Part model, mm, in its own coordinate system. A direction names the side the tool comes from. Give positions to 0.01 mm unless a question says otherwise; leave off trailing zeros. Write each loop counter-clockwise with the first axis right and the second up, starting at its lowest first coordinate (ties: lowest second). Pieces come first, ordered by that corner, then holes. Notation, with made-up numbers: M 48.25,-16 L 80.25,-16 A12 ccw 80.25,0 Z; hole C 36.5,5 d8. An arc over 180 degrees is marked long. Use CSV: the item, a comma, the result in double quotes. Start each with the question number.
1. Mould opens along Y. For faces 4 (the face through (28.71, -7.103, 0.035)), 5 (the face through (-57.15, -76.99, 0.04)), 6 (the face through (-36, -21, 27.5)) say: pulls with the +Y half, pulls with the -Y half, needs draft (parallel to the pull), parting line crosses it, or undercut.
2. Band-saw the part on C-C, the plane y = -9. List the corners of the cut face in (x, z), then the cut area to 3 significant figures.
3. Drop flat-ended pins along their axis: pin 1 Ø2 at (x, z) = (-40.5, -5) entering from -Y; pin 2 Ø5.5 at (x, z) = (-45.5, -13) entering from +Y; pin 3 Ø9 at (x, z) = (43, -10.5) entering from -Y; pin 4 Ø3.5 at (y, z) = (-59.32, -14.5) entering from -X. Give the stop position or say it passes through.
4. 3-axis set-ups, long thin cutter, end or side, ignore diameter. For faces 1 (the face through (45, -54.472, -11)), 2 (the face through (-26.29, -7.103, 0.035)), 3 (the face through (-39.064, -68.274, 14.825)): which of +Z, -Z, +X, -X, +Y, -Y reach the whole face in a straight line?
5. Drill centre lines: line 1 along Y through (x, z) = (42.5, -14.5); line 2 along Y through (x, z) = (-11, 1.5); line 3 along Z through (x, y) = (42.5, -13). Where is each one in solid material? Low to high. Write a range as from..to.
6. Band-saw the part on D-D, the plane z = -7.5. List the corners of the cut face in (x, y), then the cut area to 3 significant figures.
7. Band-saw the part on A-A, the plane z = 18. List the corners of the cut face in (x, y) (3 decimals), then the cut area to 3 significant figures.
8. Band-saw the part on B-B, the plane x = -27.5. List the corners of the cut face in (y, z), then the cut area to 4 significant figures.
from build123d import *

# Parameters (mm, degrees)
SKETCH1_W            = 120
SKETCH1_H            = 80
BOSS_EXTRUDE1_DEPTH  = 2.5
FILLET1_R            = 10
SKETCH2_R            = 2.25
CUT_EXTRUDE1_DEPTH   = 6
SKETCH3_R            = 2.5
SKETCH3_R_2          = 1.5
BOSS_EXTRUDE2_DEPTH  = 25
FILLET2_R            = 2
CUT_EXTRUDE2_DEPTH   = 2
SKETCH6_W            = 17
SKETCH6_H            = 9.5
SKETCH6_R            = 3
BOSS_EXTRUDE3_DEPTH  = 30
FILLET3_R            = 3
FILLET3_OF_MIRROR1_R = 3


with BuildPart() as part:
    # Sketch1 → Boss-Extrude1 (new body, symmetric)
    with BuildSketch(Plane.XY):
        with Locations((0, -40)):
            Rectangle(SKETCH1_W, SKETCH1_H)
    extrude(amount=BOSS_EXTRUDE1_DEPTH, both=True)

    # Fillet1
    fillet1_edges = [part.edges().sort_by_distance(p)[0] for p in [
        (60, -80, 0),
        (-60, -80, 0),
    ]]
    fillet(fillet1_edges, radius=FILLET1_R)

    # Sketch2 → Cut-Extrude1 (cut, through all)
    with BuildSketch(Plane.XY.offset(2.5)):
        with Locations((-52.5, -9)):
            Circle(SKETCH2_R)
        with Locations((-27.5, -9)):
            Circle(SKETCH2_R)
        with Locations((27.5, -9)):
            Circle(SKETCH2_R)
        with Locations((52.5, -9)):
            Circle(SKETCH2_R)
    extrude(amount=-CUT_EXTRUDE1_DEPTH, mode=Mode.SUBTRACT)

    # Sketch3 → Boss-Extrude2 (add)
    with BuildSketch(Plane.XY.offset(2.5)):
        with Locations((-37.565, -20)):
            Circle(SKETCH3_R)
        with Locations((-37.565, -20)):
            Circle(SKETCH3_R_2, mode=Mode.SUBTRACT)
        with Locations((37.565, -20)):
            Circle(SKETCH3_R)
        with Locations((37.565, -20)):
            Circle(SKETCH3_R_2, mode=Mode.SUBTRACT)
        with Locations((-37.565, -68.34)):
            Circle(SKETCH3_R)
        with Locations((-37.565, -68.34)):
            Circle(SKETCH3_R_2, mode=Mode.SUBTRACT)
        with Locations((45.065, -68.34)):
            Circle(SKETCH3_R)
        with Locations((45.065, -68.34)):
            Circle(SKETCH3_R_2, mode=Mode.SUBTRACT)
    extrude(amount=BOSS_EXTRUDE2_DEPTH)

    # Fillet2
    fillet2_edges = [part.edges().sort_by_distance(p)[0] for p in [
        (-40.065, -20, 2.5),
        (35.065, -20, 2.5),
        (-40.065, -68.34, 2.5),
        (42.565, -68.34, 2.5),
    ]]
    fillet(fillet2_edges, radius=FILLET2_R)

    # Sketch4 → Cut-Extrude2 (cut)
    with BuildSketch(Plane.XY.offset(2.5)):
        with BuildLine():
            Line((-36.5, -62), (36.5, -62))
            ThreePointArc((36.5, -62), (37.207106781, -61.707106781), (37.5, -61))
            Line((37.5, -61), (37.5, -27))
            ThreePointArc((37.5, -27), (37.207106781, -26.292893219), (36.5, -26))
            Line((36.5, -26), (-36.5, -26))
            ThreePointArc((-36.5, -26), (-37.207106781, -26.292893219), (-37.5, -27))
            Line((-37.5, -27), (-37.5, -61))
            ThreePointArc((-37.5, -61), (-37.207106781, -61.707106781), (-36.5, -62))
        make_face()
    extrude(amount=-CUT_EXTRUDE2_DEPTH, mode=Mode.SUBTRACT)

    # Sketch6 → Boss-Extrude3 (add)
    with BuildSketch(Plane(origin=(60, 0, 0), x_dir=(0, 0, -1), z_dir=(1, 0, 0))):
        with Locations((11, -59.221502787)):
            Rectangle(SKETCH6_W, SKETCH6_H)
        with Locations((14.5, -59.320826281)):
            Circle(SKETCH6_R, mode=Mode.SUBTRACT)
    boss_extrude3 = extrude(amount=-BOSS_EXTRUDE3_DEPTH)

    # Fillet3
    fillet3_edges = [part.edges().sort_by_distance(p)[0] for p in [
        (45, -54.471502787, -2.5),
        (45, -54.471502787, -19.5),
        (45, -63.971502787, -19.5),
        (45, -63.971502787, -2.5),
    ]]
    fillet(fillet3_edges, radius=FILLET3_R)

    # Mirror1: Boss-Extrude3 across plane
    add(boss_extrude3.mirror(Plane(origin=(0, 0, 0), x_dir=(0, 0, 1), z_dir=(1, 0, 0))))

    # Fillet3 of Mirror1
    fillet3_of_mirror1_edges = [part.edges().sort_by_distance(p)[0] for p in [
        (-45, -54.471502787, -2.5),
        (-45, -54.471502787, -19.5),
        (-45, -63.971502787, -19.5),
        (-45, -63.971502787, -2.5),
    ]]
    fillet(fillet3_of_mirror1_edges, radius=FILLET3_OF_MIRROR1_R)


solid = part.part
Output:
1,face 4,"undercut"
1,face 5,"pulls with the -Y half"
1,face 6,"needs draft"
2,outline,"M -60,-2.5 L -54.75,-2.5 L -54.75,2.5 L -60,2.5 Z; M -50.25,-2.5 L -29.75,-2.5 L -29.75,2.5 L -50.25,2.5 Z; M -25.25,-2.5 L 25.25,-2.5 L 25.25,2.5 L -25.25,2.5 Z; M 29.75,-2.5 L 50.25,-2.5 L 50.25,2.5 L 29.75,2.5 Z; M 54.75,-2.5 L 60,-2.5 L 60,2.5 L 54.75,2.5 Z"
2,area,"510 mm²"
3,pin 1,"stops at y = -64.37"
3,pin 2,"stops at y = -54.47"
3,pin 3,"stops at y = -63.97"
3,pin 4,"passes through"
4,face 1,"-Z, +X, -X, +Y"
4,face 2,"+Z, -Z"
4,face 3,"+Z"
5,line 1,"y = -63.97..-62.32, -56.32..-54.47"
5,line 2,"y = -80..-62, -26..0"
5,line 3,"z = -2.5..2.5"
6,outline,"M -60,-63.97 L -30,-63.97 L -30,-54.47 L -60,-54.47 Z; M 30,-63.97 L 60,-63.97 L 60,-54.47 L 30,-54.47 Z"
6,area,"570 mm²"
7,outline,"C -37.565,-68.34 d5; C -37.565,-20 d5; C 37.565,-20 d5; C 45.065,-68.34 d5; hole C -37.565,-68.34 d3; hole C -37.565,-20 d3; hole C 37.565,-20 d3; hole C 45.065,-68.34 d3"
7,area,"50.3 mm²"
8,outline,"M -80,-2.5 L -11.25,-2.5 L -11.25,2.5 L -26,2.5 L -26,0.5 L -62,0.5 L -62,2.5 L -80,2.5 Z; M -6.75,-2.5 L 0,-2.5 L 0,2.5 L -6.75,2.5 Z"
8,area,"305.5 mm²"
